Build history of the part. All positions in model axes, mm. A direction names the side the tool comes from. Round coordinates to 2 decimals unless told otherwise and drop trailing zeros. Loops run counter-clockwise (first coordinate to the right, second up) from the corner with the lowest first, then second, coordinate; pieces in that order, holes last. Notation, with made-up numbers: (41.5, 36) -> (57.5, 36) arc R25 cw to (57.5, 60) -> close; hole circle Ø3 at (-11.75, 4). An arc over 180 degrees is marked (long way). Put each result on its own line as item: value. Start each with the question number.
```python
from build123d import *

# Parameters (mm, degrees)
F1_DEPTH = 76.2
F4_DEPTH = 2.54
F5_T     = -2.54
F6_R     = 7.62


# Not quite as in the source:
# - a shell that OpenCascade refuses in one call is made with other operations: the cavity is built on its own and cut out


with BuildPart() as f1:
    # F0 (on Top) → F1 (new body)
    with BuildSketch(Plane.XY):
        Polygon((0, -69.1435125567), (0, 74.5809290344), (-50.8, 47.6656096473), (-50.8, -42.2281931696), align=None)
        Polygon((50.8, 47.6656096473), (0, 74.5809290344), (0, -69.1435125567), (50.8, -42.2281931696), align=None)
    extrude(amount=F1_DEPTH)

    # F3 (on offset) → F4 (join)
    with BuildSketch(Plane.XY.offset(76.2)):
        Polygon((76.2, 47.5584119558), (0, 110.1294793168), (-76.2, 47.5584119558), (-76.2, -42.4090027809), (0, -101.7426550388), (76.2, -42.4090027809), align=None)
        Polygon((-49.5749972761, 47.5584119558), (0, 72.8662833571), (49.6499985456, 47.5584119558), (49.6499985456, -42.4090027809), (0, -67.1015977859), (-49.5749972761, -42.4090027809), align=None, mode=Mode.SUBTRACT)
    extrude(amount=F4_DEPTH)

    # F5: a shell. OpenCascade refuses it in one call, so the cavity is built on its own and cut out:
    # the body offset inwards by the wall thickness, plus a prism from it out through each open face.
    f5_core = offset(f1.part, amount=F5_T, mode=Mode.PRIVATE)
    f5_exits = [f5_core.faces().sort_by_distance(p)[0] for p in [
        (0, 2.718708, 73.66),
    ]]
    add(f5_core, mode=Mode.SUBTRACT)
    extrude(f5_exits, amount=-F5_T, mode=Mode.SUBTRACT)

    # F6
    f6_edges = [f1.edges().sort_by_distance(p)[0] for p in [
        (-25.4, 61.123269, 0),
        (-50.8, 2.718708, 0),
        (-25.4, -55.685853, 0),
        (25.4, -55.685853, 0),
        (50.8, 2.718708, 0),
        (25.4, 61.123269, 0),
    ]]
    fillet(f6_edges, radius=F6_R)


solid = f1.part
```
Item 1: Cut at C-C on x = -61. Write the cut outline in (y, z), then the cut area to 3 significant figures.
Item 2: Pull direction Y, two halves, no side cores. Call faces 1 (the face through (24.68, -53.47, 2.17)), 2 (the face through (24.03, 59.39, 2.29)), 3 (the face through (-25.135, 60.035, 77.452)): +Y half, -Y half, draft (parallel to the pull), parting line (faces both ways), or undercut.
Item 3: Cut at D-D on y = 95. Write the cut outline in (x, z), then the cut area to 3 significant figures.
Item 4: Cut at A-A on z = 23.5. Write the cut outline in (x, y), then the cut area to 3 significant figures.
Item 5: Cut at B-B on y = 17. Write the cut outline in (x, z) (3 decimals).
Item 6: Drop flat-ended pins along their axis: pin 1 (5 mm diameter, centred on y = -1.5, z = 10.5, fed in from -X); pin 2 (1.5 mm diameter, centred on y = 13, z = 62, fed in from +X); pin 3 (10 mm diameter, centred on x = 44.5, z = 59.5, fed in from -Y). Give the stop position or say it passes through.
Item 7: 3-axis set-ups, long thin cutter, end or side, ignore diameter. For faces 4 (the face through (-25.044, 61.312, 41.43)), 5 (the face through (25.756, 60.935, 41.43)), 6 (the face through (48.26, 3, 39)): which of +Z, -Z, +X, -X, +Y, -Y reach the whole face in a straight line?
Item 8: Wall check: line 1 (X direction, y = -22.5, z = 34); line 2 (Z direction, x = -37, y = 63); line 3 (Y direction, x = -10, z = 56). Give the ranges that are in metal, low to high. Write a range as from..to.
Ans:
1. outline: (-54.24, 76.2) -> (60.04, 76.2) -> (60.04, 78.74) -> (-54.24, 78.74) -> close
1. area: 290 mm2
2. face 1: -Y half
2. face 2: +Y half
2. face 3: undercut
3. outline: (-18.42, 76.2) -> (18.42, 76.2) -> (18.42, 78.74) -> (-18.42, 78.74) -> close
3. area: 93.6 mm2
4. outline: (-50.8, -42.23) -> (0, -69.14) -> (50.8, -42.23) -> (50.8, 47.67) -> (0, 74.58) -> (-50.8, 47.67) -> close; hole (-48.26, -40.7) -> (0, -66.27) -> (48.26, -40.7) -> (48.26, 46.14) -> (0, 71.71) -> (-48.26, 46.14) -> close
4. area: 1,020 mm2
5. outline: (-76.2, 76.2) -> (-50.8, 76.2) -> (-50.8, 7.62) arc R7.62 ccw to (-43.18, 0) -> (43.18, 0) arc R7.62 ccw to (50.8, 7.62) -> (50.8, 76.2) -> (76.2, 76.2) -> (76.2, 78.74) -> (49.65, 78.74) -> (49.65, 76.2) -> (48.26, 76.2) -> (48.26, 2.54) -> (-48.26, 2.54) -> (-48.26, 76.2) -> (-49.575, 76.2) -> (-49.575, 78.74) -> (-76.2, 78.74) -> close
6. pin 1: stops at x = -50.8
6. pin 2: stops at x = 50.8
6. pin 3: stops at y = -48.22
7. face 4: -Z, -X, +Y
7. face 5: -Z, +X, +Y
7. face 6: +Z
8. line 1: x = -50.8..-48.26, 48.26..50.8
8. line 2: z = 76.2..78.74
8. line 3: y = -63.85..-60.97, 66.41..69.28
